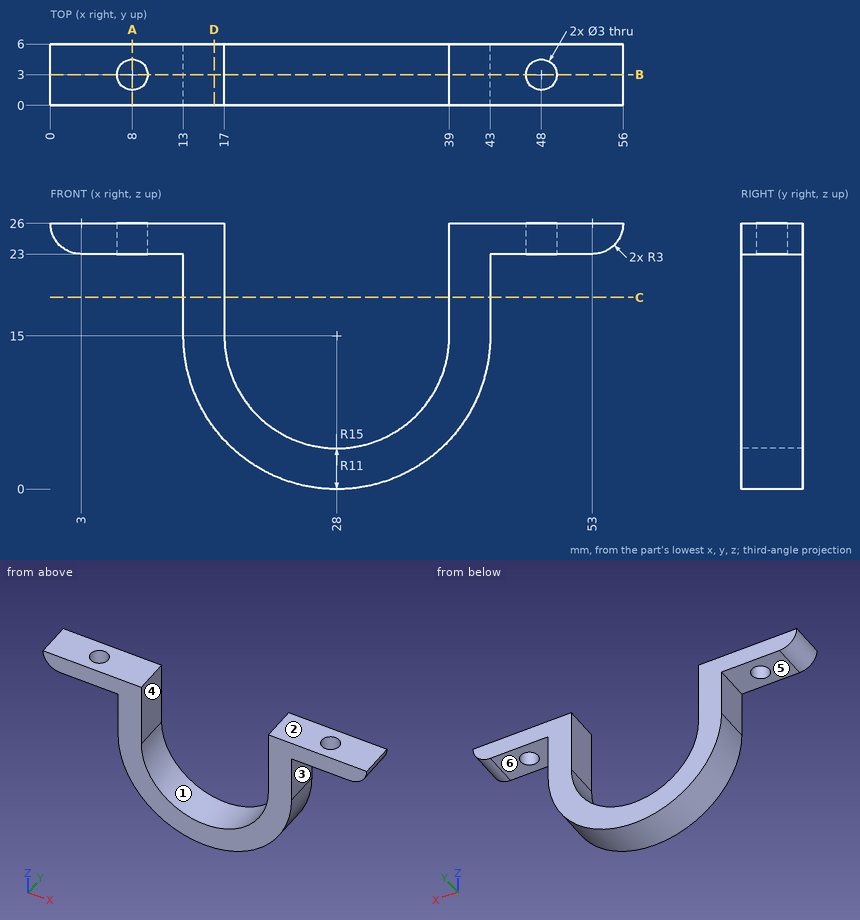
Geometry: see drawing. Coordinates: mm, zero at the bounding-box minimum. A direction names the side the tool comes from. Round coordinates to 2 decimals unless told otherwise and drop trailing zeros. Write each loop counter-clockwise with the first axis right and the second up, starting at its lowest first coordinate (ties: lowest second). Pieces come first, ordered by that corner, then holes.
Item 1: Section query B-B (y = 3). Return loops of the section in (x, z).
Item 2: Material intervals for L1, parallel to Y at x = 8, z = 24.3; L2, parallel to X at y = 0.65, z = 16.75; L3, parallel to X at y = 4.15, z = 24, sorted ascending.
Item 3: Section query A-A (x = 8). Return loops of the section in (y, z), plus the area to 3 significant figures.
Item 4: Set-up query: the marked faces 4, 5 and 6. Return all of +Z, -Z, +X, -X, +Y, -Y with unobstructed straight access to the full face (end or side cutting, diameter ignored); none if empty.
Item 5: Section query D-D (x = 16). Return loops of the section in (y, z), plus the area to 3 significant figures.
Item 6: Pin query (flat end, axial travel): P1, Ø1.8, axis at y = 2.5, z = 20, coming from the -X side; P2, Ø6, axis at x = 23, z = 10.5, coming from the -Y side (3 decimals); P3, Ø2, axis at y = 3.5, z = 11, coming from the +X side; P4, Ø1.8, axis at x = 5.5, y = 3.5, coming from the -Z side. Return the tip coordinate at first contact, or that it passes through.
Item 7: Section query C-C (z = 18.75). Return loops of the section in (x, y), plus the area to 3 significant figures.
Item 8: Mould query, pull axis X, two halves, no side actions, for the marked faces 1, 2 and 3. Classes: +X half, -X half, draft (parallel to the pull), parting line (faces both ways), or undercut.
Completed:
1. outline: (0, 26) arc R3 ccw to (3, 23) - (6.5, 23) - (6.5, 26) - close; (9.5, 23) - (13, 23) - (13, 15) arc R15 ccw to (43, 15) - (43, 23) - (46.5, 23) - (46.5, 26) - (39, 26) - (39, 15) arc R11 cw to (17, 15) - (17, 26) - (9.5, 26) - close; (49.5, 23) - (53, 23) arc R3 ccw to (56, 26) - (49.5, 26) - close
2. L1: y = 0 to 1.5, 4.5 to 6
2. L2: x = 13 to 17, 39 to 43
2. L3: x = 0.76 to 7.04, 8.96 to 17, 39 to 47.04, 48.96 to 55.24
3. outline: (0, 23) - (1.5, 23) - (1.5, 26) - (0, 26) - close; (4.5, 23) - (6, 23) - (6, 26) - (4.5, 26) - close
3. area: 9.00 mm2
4. face 4: +Z, +Y, -Y
4. face 5: -Z, -X, +Y, -Y
4. face 6: -Z, +X, +Y, -Y
5. outline: (0, 6) - (6, 6) - (6, 26) - (0, 26) - close
5. area: 120 mm2
6. P1: stops at x = 13
6. P2: passes through
6. P3: stops at x = 42.7
6. P4: stops at z = 23
7. outline: (13, 0) - (17, 0) - (17, 6) - (13, 6) - close; (39, 0) - (43, 0) - (43, 6) - (39, 6) - close
7. area: 48.0 mm2
8. face 1: undercut
8. face 2: draft
8. face 3: +X half
